The model under review builds one solid part; all positions refer to its coordinate system, in mm. Face numbers are marked on the shaded views. Coordinates: 2 decimals unless noted, no trailing zeros. Order: outer loops, then holes, each group sorted by start corner. A loop starts at its lowest first (then second) coordinate and runs counter-clockwise, first axis right, second up. Notation, with made-up numbers: (-5.75, 57) -> (34.25, 57) arc R25 ccw to (34.25, 91) -> close; hole circle Ø7 at (63, 80.5). An arc over 180 degrees is marked (long way). Use one line per item in the form item = value.
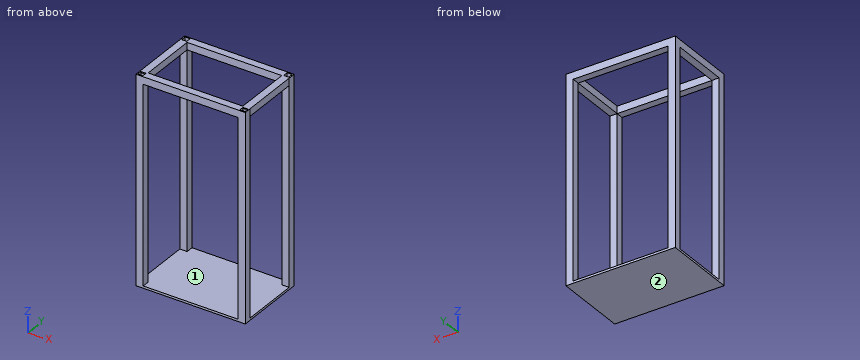
from build123d import *

# Parameters (mm, degrees)
SKETCH1_W           = 150
SKETCH1_H           = 100
BOSS_EXTRUDE1_DEPTH = 3
SKETCH2_W           = 10
SKETCH2_H           = 10
SKETCH2_W_2         = 7
SKETCH2_H_2         = 7
BOSS_EXTRUDE2_DEPTH = 280
SKETCH3_W           = 10
SKETCH3_H           = 10
SKETCH3_W_2         = 7
SKETCH3_H_2         = 7
BOSS_EXTRUDE3_DEPTH = 130
SKETCH4_W           = 10
SKETCH4_H           = 10
SKETCH4_W_2         = 7
SKETCH4_H_2         = 7
BOSS_EXTRUDE4_DEPTH = 130
SKETCH5_W           = 10
SKETCH5_H           = 10
SKETCH5_W_2         = 7
SKETCH5_H_2         = 7
BOSS_EXTRUDE5_DEPTH = 82


with BuildPart() as part:
    # Sketch1 → Boss-Extrude1 (new body)
    with BuildSketch(Plane.XY):
        with Locations((75, 50)):
            Rectangle(SKETCH1_W, SKETCH1_H)
    extrude(amount=BOSS_EXTRUDE1_DEPTH)

    # Sketch2 → Boss-Extrude2 (add)
    # profile 1 of 4: a face of its own
    with BuildSketch(Plane.XY.offset(3)):
        with Locations((145, 95)):
            Rectangle(SKETCH2_W, SKETCH2_H)
        with Locations((145, 95)):
            Rectangle(SKETCH2_W_2, SKETCH2_H_2, mode=Mode.SUBTRACT)
    # profile 2 of 4: a face of its own
    with BuildSketch(Plane.XY.offset(3)):
        with Locations((145, 5)):
            Rectangle(SKETCH2_W, SKETCH2_H)
        with Locations((145, 5)):
            Rectangle(SKETCH2_W_2, SKETCH2_H_2, mode=Mode.SUBTRACT)
    # profile 3 of 4: a face of its own
    with BuildSketch(Plane.XY.offset(3)):
        with Locations((5, 5)):
            Rectangle(SKETCH2_W, SKETCH2_H)
        with Locations((5, 5)):
            Rectangle(SKETCH2_W_2, SKETCH2_H_2, mode=Mode.SUBTRACT)
    # profile 4 of 4: a face of its own
    with BuildSketch(Plane.XY.offset(3)):
        with Locations((5, 95)):
            Rectangle(SKETCH2_W, SKETCH2_H)
        with Locations((5, 95)):
            Rectangle(SKETCH2_W_2, SKETCH2_H_2, mode=Mode.SUBTRACT)
    extrude(amount=BOSS_EXTRUDE2_DEPTH)

    # Sketch3 → Boss-Extrude3 (add)
    with BuildSketch(Plane.ZY.offset(-140)):
        with Locations((278, 95)):
            Rectangle(SKETCH3_W, SKETCH3_H)
        with Locations((278, 95)):
            Rectangle(SKETCH3_W_2, SKETCH3_H_2, mode=Mode.SUBTRACT)
    extrude(amount=BOSS_EXTRUDE3_DEPTH)

    # Sketch4 → Boss-Extrude4 (add)
    with BuildSketch(Plane.ZY.offset(-140)):
        with Locations((278, 5)):
            Rectangle(SKETCH4_W, SKETCH4_H)
        with Locations((278, 5)):
            Rectangle(SKETCH4_W_2, SKETCH4_H_2, mode=Mode.SUBTRACT)
    extrude(amount=BOSS_EXTRUDE4_DEPTH)

    # Sketch5 → Boss-Extrude5 (add)
    # profile 1 of 2: a face of its own
    with BuildSketch(Plane.XZ.offset(-90)):
        with Locations((5, 278)):
            Rectangle(SKETCH5_W, SKETCH5_H)
        with Locations((5, 278)):
            Rectangle(SKETCH5_W_2, SKETCH5_H_2, mode=Mode.SUBTRACT)
    # profile 2 of 2: a face of its own
    with BuildSketch(Plane.XZ.offset(-90)):
        with Locations((144.9, 278)):
            Rectangle(SKETCH5_W, SKETCH5_H)
        with Locations((144.9, 278)):
            Rectangle(SKETCH5_W_2, SKETCH5_H_2, mode=Mode.SUBTRACT)
    extrude(amount=BOSS_EXTRUDE5_DEPTH)


solid = part.part
Item 1: We need section B-B (x = 118.5). Write out the cut boundary in (y, z).
Results found:
outline = (0, 0) -> (100, 0) -> (100, 3) -> (0, 3) -> close; (0, 273) -> (10, 273) -> (10, 283) -> (0, 283) -> close; (90, 273) -> (100, 273) -> (100, 283) -> (90, 283) -> close; hole (1.5, 274.5) -> (8.5, 274.5) -> (8.5, 281.5) -> (1.5, 281.5) -> close; hole (91.5, 274.5) -> (98.5, 274.5) -> (98.5, 281.5) -> (91.5, 281.5) -> close
Item 2: Clearance check with flat-ended pins moving along their axes: pin 1 (8 mm diameter, centred on x = 58.5, y = 59.5, fed in from +Z); pin 2 (5 mm diameter, centred on x = 79.5, z = 279.5, fed in from -Y); pin 3 (3 mm diameter, centred on y = 36.5, z = 277.5, fed in from +X). State where each tip first meets the part, or that it passes through.
Results found:
pin_1 = 3
pin_2 = 0
pin_3 = 149.9
Item 3: To check wall thickness, follow L1, parallel to Z at x = 8, y = 24; L2, parallel to Z at x = 102, y = 52.5. State the ranges of each line that lie inside material, in increasing order. Write a range as from..to.
Results found:
L1 = 0..3, 273..274.5, 281.5..283
L2 = 0..3
Item 4: We need section A-A (y = 87). Write out the cut boundary in (x, z), plus the area to 3 significant figures.
Results found:
outline = (0, 0) -> (150, 0) -> (150, 3) -> (0, 3) -> close; (0, 273) -> (10, 273) -> (10, 283) -> (0, 283) -> close; (139.9, 273) -> (149.9, 273) -> (149.9, 283) -> (139.9, 283) -> close; hole (1.5, 274.5) -> (8.5, 274.5) -> (8.5, 281.5) -> (1.5, 281.5) -> close; hole (141.4, 274.5) -> (148.4, 274.5) -> (148.4, 281.5) -> (141.4, 281.5) -> close
area = 552 mm²
Item 5: We need section C-C (z = 85). State how many separate pieces and enclosed holes the cut face has, plus the area to 3 significant figures.
Results found:
separate_pieces = 4
enclosed_holes = 4
area = 204 mm²
Item 6: Draft analysis for pull direction X (two halves, no side actions). For the marked faces 1 and 2, state which applies: released by +X, released by -X, zero draft, split by the parting line, or undercut.
Results found:
face_1 = undercut
face_2 = zero draft
